Autodesk Inventor part; units mm, degrees
ref_plane "YZ Plane" through (0, 0, 0) normal (1, 0, 0) x (0, 1, 0)
ref_plane "XZ Plane" through (0, 0, 0) normal (0, 1, 0) x (-1, 0, 0)
ref_plane "XY Plane" through (0, 0, 0) normal (0, 0, 1) x (1, 0, 0)
sketch "Sketch1" plane through (0, 0, 0) normal (1, 0, 0) x (0, 1, 0)
  line L0 (0, 0) -> (51, 0)
  line L1 (51, 0) -> (51, 2)
  line L2 (51, 2) -> (0, 2)
  line L3 (-2, 0) -> (-2, -51)
  line L4 (-2, -51) -> (0, -51)
  line L5 (0, -51) -> (0, 0)
  line L6 (0, 0) -> (-2, 0)
  line L7 (-2, 0) -> (-2, 2)
  line L8 (-2, 2) -> (0, 2)
  line L9 (0, 2) -> (0, 0)
  dimension "d0" = 51
  dimension "d1" = 2
  dimension "d2" = 2
  dimension "d3" = 51
extrude "Extrusion1" add sketch "Sketch1" along normal blind 50
sketch "Sketch2" plane through (0, 0, 0) normal (0, 0, -1) x (-1, 0, 0)
  line L0 (0, 51) -> (-50, 51)
  line L1 (-25, 51) -> (-25, 30)
  circle A0 centre (-25, 30) radius 6.5
  line L2 (-25, 51) -> (-9.5, 51)
  line L3 (-25, 30) -> (-9.5, 30)
  line L4 (-9.5, 30) -> (-9.5, 45.5)
  line L5 (-9.5, 30) -> (-9.5, 14.5)
  circle A1 centre (-9.5, 14.5) radius 2
  circle A2 centre (-9.5, 45.5) radius 2
  circle A3 centre (-40.5, 14.5) radius 2
  circle A4 centre (-40.5, 45.5) radius 2
  point P0 (0, 0)
  dimension "d6" = 21
  dimension "d7" = 13
  dimension "d8" = 15.5
  dimension "d9" = 15.5
  dimension "d10" = 15.5
  dimension "d11" = 4
  dimension "d12" = 4
extrude "Extrusion2" cut sketch "Sketch2" against normal blind 50
sketch "Sketch3" plane through (0, 0, 0) normal (0, 1, 0) x (1, 0, 0)
  line L0 (0, 51) -> (50, 51)
  line L1 (25, 51) -> (25, 36)
  line L2 (25, 36) -> (25, 13)
  circle A0 centre (25, 13) radius 3
  circle A1 centre (25, 36) radius 3
  point P0 (0, 0)
  dimension "d15" = 15
  dimension "d16" = 23
  dimension "d17" = 6
  dimension "d18" = 6
extrude "Extrusion3" cut sketch "Sketch3" against normal blind 50
sketch "Sketch4" plane through (0, -2, 2) normal (0, 0, 1) x (1, 0, 0)
  circle A0 centre (25, 32) radius 6.5
  circle A1 centre (25, 32) radius 7.5
  circle A2 centre (25, 32) radius 6.5
  point P0 (0, 2)
  dimension "d21" = 15
extrude "Extrusion4" add sketch "Sketch4" along normal blind 5
properties part number "NEMA17-3030-m6-holder" material "Aluminum 6061"
Input: part model. Units: mm. Frame: model coordinates. A direction names the side the tool comes from. Round coordinates to 2 decimals unless told otherwise and drop trailing zeros. Order: outer loops, then holes, each group sorted by start corner. A loop starts at its lowest first (then second) coordinate and runs counter-clockwise, first axis right, second up. Notation, with made-up numbers: (35, 48) - (50, 48) arc R14 cw to (50, 55) - close; hole circle Ø9 at (75.25, 85). An arc over 180 degrees is marked (long way). Answer as a JSON object with one key per item and string values. Group by question number.
(1) Pin query (flat end, axial travel): P1, Ø7, axis at x = 25, z = -13, coming from the +Y side; P2, Ø6.5, axis at x = 40.5, y = 14.5, coming from the +Z side; P3, Ø3, axis at x = 22.5, y = 6.5, coming from the -Z side; P4, Ø3.5, axis at x = 25, z = -36, coming from the +Y side. Return the tip coordinate at first contact, or that it passes through.
(2) Material intervals for probe 1 along Y at (x, z) = (40.5, 0.65); probe 2 along Y at (x, z) = (25, 2.5); probe 3 along Z at (x, y) = (48, 44.5), sorted ascending. Write a range as from..to.
(3) Cut plane B-B (z = -13). Return loops of the section in (x, y).
(4) Draft query along Y for faces 4 (the face through (25, -1, -51)), 5 (the face through (25, 51, 1)), 6 (the face through (8.577, 43.726, 0.986)). Return one class per face: released by +Y, released by -Y, zero draft, split by the parting line, or undercut.
(5) Cut plane D-D (x = 25). Return loops of the section in (y, z).
(6) Cut plane C-C (y = 30). Return loops of the section in (x, z).
(7) Cut plane A-A (x = 9.5). Return loops of the section in (y, z).
(8) Reachability of faces 1 (the face through (19.048, 34.564, 4.465)), 2 (the face through (19, 25, 0)), 3 (the face through (40.934, 43.548, 0.986)) from +Z, -Z, +X, -X, +Y, -Y: full face, straight path, thin tool, end or side. Return the list, or none.
Here are the results:
{
 "1": {"P1": "stops at y = 0", "P2": "stops at z = 2", "P3": "stops at z = 0", "P4": "passes through"},
 "2": {"probe 1": "y = -2..12.5, 16.5..43.5, 47.5..51", "probe 2": "y = 22.5..23.5, 36.5..37.5", "probe 3": "z = 0..2"},
 "3": {"outline": "(0, -2) - (22, -2) - (22, 0) - (0, 0) - close; (28, -2) - (50, -2) - (50, 0) - (28, 0) - close"},
 "4": {"face 4": "zero draft", "face 5": "released by +Y", "face 6": "undercut"},
 "5": {"outline": "(-2, -51) - (0, -51) - (0, -39) - (-2, -39) - close; (-2, -33) - (0, -33) - (0, -16) - (-2, -16) - close; (-2, -10) - (0, -10) - (0, 0) - (23.5, 0) - (23.5, 7) - (22.5, 7) - (22.5, 2) - (-2, 2) - close; (36.5, 0) - (51, 0) - (51, 2) - (37.5, 2) - (37.5, 7) - (36.5, 7) - close"},
 "6": {"outline": "(0, 0) - (18.5, 0) - (18.5, 7) - (17.5, 7) - (17.5, 2) - (0, 2) - close; (31.5, 0) - (50, 0) - (50, 2) - (32.5, 2) - (32.5, 7) - (31.5, 7) - close"},
 "7": {"outline": "(-2, -51) - (0, -51) - (0, 0) - (12.5, 0) - (12.5, 2) - (-2, 2) - close; (16.5, 0) - (43.5, 0) - (43.5, 2) - (16.5, 2) - close; (47.5, 0) - (51, 0) - (51, 2) - (47.5, 2) - close"},
 "8": {"face 1": "+Z", "face 2": "-Z, +X, -X, +Y", "face 3": "+Z, -Z"}
}
